```python
from build123d import *

# Parameters (mm, degrees)
CHAMFER1_SIZE      = 0.8
CUT_EXTRUDE1_DEPTH = 4


with BuildPart() as part:
    # Sketch1 → Revolve1 (revolve)
    with BuildSketch(Plane.XY):
        Polygon((-8, 0), (-8, 6.5), (0, 6.5), (0, 4), (20, 4), (20, 0), align=None)
    revolve(axis=Axis((20, 0, 0), (-1, 0, 0)))

    # Chamfer1
    chamfer1_edges = [part.edges().sort_by_distance(p)[0] for p in [
        (20, -4, 0),
        (-8, -6.5, 0),
    ]]
    chamfer(chamfer1_edges, length=CHAMFER1_SIZE)

    # Sketch2 → Cut-Revolve1 (revolve, cut)
    with BuildSketch(Plane.XY):
        Polygon((-8, 0), (-8, 3), (-4, 3), (-3.196152423, 0), align=None)
    revolve(axis=Axis((-3.196152423, 0, 0), (-1, 0, 0)), mode=Mode.SUBTRACT)

    # Sketch3 → Cut-Extrude1 (cut)
    with BuildSketch(Plane(origin=(-8, 0, 0), x_dir=(0, 0, -1), z_dir=(1, 0, 0))):
        Polygon((-3, 1.732050808), (-3, -1.732050808), (0, -3.464101615), (3, -1.732050808), (3, 1.732050808), (0, 3.464101615), align=None)
    extrude(amount=CUT_EXTRUDE1_DEPTH, mode=Mode.SUBTRACT)


solid = part.part
```
Part model, mm, in its own coordinate system. A direction names the side the tool comes from. Round coordinates to 2 decimals unless told otherwise and drop trailing zeros. Loops run counter-clockwise (first coordinate to the right, second up) from the corner with the lowest first, then second, coordinate; pieces in that order, holes last.
Item 1: Drop flat-ended pins along their axis: P1, Ø0.8, axis at y = 1, z = 2.5, coming from the -X side; P2, Ø1.5, axis at x = 9, y = -1, coming from the -Z side; P3, Ø1.5, axis at x = 6.5, z = -0.5, coming from the +Y side. Give the stop position or say it passes through.
Item 2: Cut at A-A, the plane x = -4.75. Give the cut face in (y, z), then the cut area to 3 significant figures.
Item 3: Mould opens along Y. For faces 3 (the face through (20, 0, 0)), 4 (the face through (-4, 1.59, -2.75)), 5 (the face through (-3.55, -5.158, 3.955)) say: +Y half, -Y half, draft (parallel to the pull), parting line (faces both ways), or undercut.
Item 4: Cut at C-C, the plane x = 11. Give the cut face in (y, z), then the cut area to 3 significant figures.
Item 5: Cut at B-B, the plane x = -0.5. Give the cut face in (y, z), then the cut area to 3 significant figures.
Item 6: 3-axis set-ups, long thin cutter, end or side, ignore diameter. For faces 1 (the face through (-6, -2.6, 1.5)), 2 (the face through (9.734, -0.867, 3.905)): which of +Z, -Z, +X, -X, +Y, -Y reach the whole face in a straight line?
Item 7: Drill centre lines: line 1 (Z direction, x = 9, y = 0); line 2 (X direction, y = -4.5, z = 2.5); line 3 (X direction, y = -2, z = 2.25). Where is each one in solid material? Low to high.
A:
1. P1: stops at x = -4
1. P2: stops at z = -3.99
1. P3: stops at y = 4
2. outline: circle Ø13 at (0, 0); hole (-3.46, 0) - (-1.73, -3) - (1.73, -3) - (3.46, 0) - (1.73, 3) - (-1.73, 3) - close
2. area: 102 mm2
3. face 3: draft
3. face 4: undercut
3. face 5: parting line
4. outline: circle Ø8 at (0, 0)
4. area: 50.3 mm2
5. outline: circle Ø13 at (0, 0)
5. area: 133 mm2
6. face 1: -X
6. face 2: +X
7. line 1: z = -4 to 4
7. line 2: x = -8 to 0
7. line 3: x = -4 to 20
